Autodesk Inventor part; units mm, degrees
ref_plane "YZ Plane" through (0, 0, 0) normal (1, 0, 0) x (0, 1, 0)
ref_plane "XZ Plane" through (0, 0, 0) normal (0, 1, 0) x (-1, 0, 0)
ref_plane "XY Plane" through (0, 0, 0) normal (0, 0, 1) x (1, 0, 0)
sketch "Sketch1" plane through (0, 0, 0) normal (0, 1, 0) x (-1, 0, 0)
  line L0 (60, 12.5) -> (-60, 12.5)
  line L1 (-60, 12.5) -> (-60, -12.5)
  line L2 (-60, -12.5) -> (60, -12.5)
  line L3 (60, -12.5) -> (60, 12.5)
  line L4 (60, 12.5) -> (-60, -12.5) construction
  line L5 (-60, 12.5) -> (60, -12.5) construction
  point P0 (0, 0)
  dimension "d0" = 120
  dimension "d1" = 25
extrude "Extrusion1" add sketch "Sketch1" along normal blind 5
sketch "Sketch2" plane through (0, 5, 0) normal (0, 1, 0) x (1, 0, 0)
  circle A0 centre (-50.0145, 0) radius 3.5
  circle A1 centre (-34.0609, 0) radius 3.5
  point P0 (0, 0)
  dimension "d4" = 7
  dimension "d5" = 7
extrude "Extrusion2" cut sketch "Sketch2" against normal blind 20
sketch "Sketch3" plane through (0, 5, 0) normal (0, 1, 0) x (1, 0, 0)
  circle A0 centre (50.148, 0) radius 1.5
  point P0 (0, 0)
  dimension "d8" = 3
extrude "Extrusion3" cut sketch "Sketch3" against normal blind 20
properties part number "Stationary arm 2"
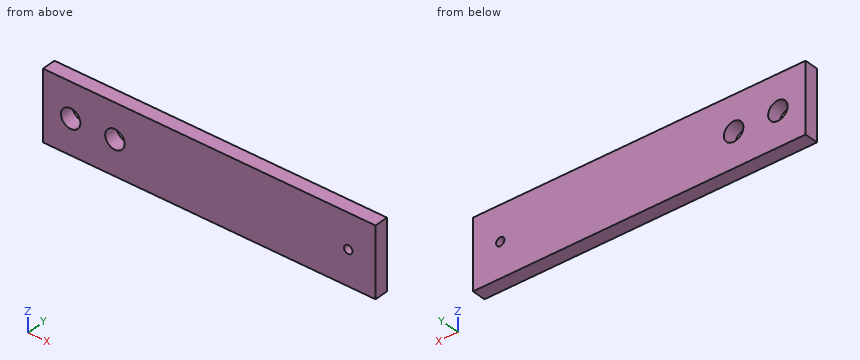
Geometry check sheet. Reference: the model listing, model coordinates, mm. Round coordinates to 2 decimals unless told otherwise and drop trailing zeros. Write each loop counter-clockwise with the first axis right and the second up, starting at its lowest first coordinate (ties: lowest second). Pieces come first, ordered by that corner, then holes.
Item 1: Section check B-B (x = -48.5). Record the boundary of the cut face in (y, z), plus the area to 3 significant figures.
Determined:
outline: (0, -12.5) - (5, -12.5) - (5, -3.16) - (0, -3.16) - close; (0, 3.16) - (5, 3.16) - (5, 12.5) - (0, 12.5) - close
area: 93.4 mm2
Item 2: Material ranges on line 1 along X through (y, z) = (2.45, 0); line 2 along X through (y, z) = (1.5, 1.75); line 3 along X through (y, z) = (4.55, 0.5) (3 decimals), recorded low to high.
Determined:
line 1: x = -60 to -53.51, -46.51 to -37.56, -30.56 to 48.65, 51.65 to 60
line 2: x = -60 to -53.05, -46.98 to -37.09, -31.03 to 60
line 3: x = -60 to -53.479, -46.55 to -37.525, -30.597 to 48.734, 51.562 to 60
Item 3: Go/stop test with flat-tipped pins: pin 1 Ø5 at (x, z) = (-32, -6) entering from -Y; pin 2 Ø6.5 at (x, z) = (-34.06, 0) entering from +Y. Record where each tip stops, or that it passes through.
Determined:
pin 1: stops at y = 0
pin 2: passes through
Item 4: Section check A-A (z = 0). Record the boundary of the cut face in (x, y).
Determined:
outline: (-60, 0) - (-53.51, 0) - (-53.51, 5) - (-60, 5) - close; (-46.51, 0) - (-37.56, 0) - (-37.56, 5) - (-46.51, 5) - close; (-30.56, 0) - (48.65, 0) - (48.65, 5) - (-30.56, 5) - close; (51.65, 0) - (60, 0) - (60, 5) - (51.65, 5) - close
Item 5: Section check C-C (y = 1.4). Record the boundary of the cut face in (x, z), plus the area to 3 significant figures.
Determined:
outline: (-60, -12.5) - (60, -12.5) - (60, 12.5) - (-60, 12.5) - close; hole circle Ø7 at (-50.01, 0); hole circle Ø7 at (-34.06, 0); hole circle Ø3 at (50.15, 0)
area: 2,920 mm2
